Could you check a few things on this model? Use its own coordinates, in mm. Face numbers are marked on the shaded views. A direction names the side the tool comes from. Round coordinates to 2 decimals unless told otherwise and drop trailing zeros. Order: outer loops, then holes, each group sorted by start corner. A loop starts at its lowest first (then second) coordinate and runs counter-clockwise, first axis right, second up. Notation, with made-up numbers: (35.5, 49.25) - (44.5, 49.25) arc R28 cw to (44.5, 83.25) - close; hole circle Ø5 at (86.25, 89.25). An arc over 180 degrees is marked (long way). Return JSON: item names as keys, results as strings. Group by question number.
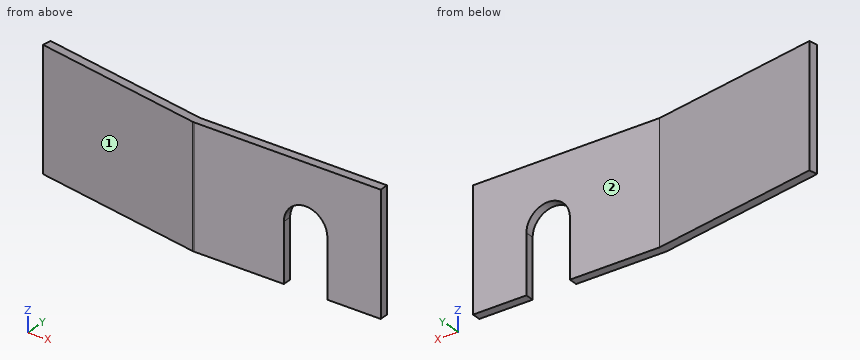
from build123d import *

# Parameters (mm, degrees)
F1_DEPTH      = 3
F3_DEPTH      = 21.6650813818
F3_DEPTH_BACK = 20.2457859941


with BuildPart() as f1:
    # F0 (on Front) → F1 (new body)
    with BuildSketch(Plane.XZ):
        with BuildLine():
            ThreePointArc((-7.5, 0), (0, 7.5), (7.5, 0))
            Line((7.5, 0), (7.5, -20.2457859941))
            Line((7.5, -20.2457859941), (25.9074462614, -20.2457859941))
            Line((25.9074462614, -20.2457859941), (25.9074462614, 21.6650813818))
            Line((25.9074462614, 21.6650813818), (-38.4318618068, 21.6650813818))
            Line((-38.4318618068, 21.6650813818), (-38.4318618068, -20.2457859941))
            Line((-38.4318618068, -20.2457859941), (-7.5, -20.2457859941))
            Line((-7.5, -20.2457859941), (-7.5, 0))
        make_face()
    extrude(amount=F1_DEPTH)

    # F2 (on Top) → F3 (join, two sides)
    with BuildSketch(Plane.XY) as f3_sk:
        with BuildLine():
            Line((-38.4318618068, -3), (-38.4318618068, 0))
            Line((-38.4318618068, 0), (-97.5203269875, 10.41889066))
            Line((-97.5203269875, 10.41889066), (-98.0412715205, 7.464467401))
            Line((-98.0412715205, 7.464467401), (-38.9528063398, -2.954423259))
            ThreePointArc((-38.9528063398, -2.954423259), (-38.693329035, -2.9885840943), (-38.4318618068, -3))
        make_face()
    extrude(amount=F3_DEPTH)
    extrude(f3_sk.sketch, amount=-F3_DEPTH_BACK)


solid = f1.part
1) If I drill on line 1 along Y through (x, z) = (18, 13.5); line 2 along Y through (x, z) = (-39.5, -15), over which ranges is the centre line in solid material (lowest first)? Write a range as from..to.
2) I want a section at B-B, the plane z = 18. List the corners of the cut face in (x, y) for me.
3) I want a section at D-D, the plane x = 0. List the corners of the cut face in (y, z) for me.
4) Will these pins go through, and if not, where does the flat tip stop? pin 1 (5 mm diameter, centred on x = -32.5, z = -1, fed in from +Y); pin 2 (1 mm diameter, centred on x = -80.5, y = 3, fed in from -Z).
5) For the marked faces 1 and 2, which set-ups out of +Z, -Z, +X, -X, +Y, -Y let a thin tool reach every point of the face, with its end or its side?
6) I want a section at C-C, the plane y = -1.25. List the corners of the cut face in (x, z) for me.
7) I want a section at A-A, the plane z = -17. List the corners of the cut face in (x, y) for me, plus the area to 3 significant figures.
Outcome:
{
 "1": {"line 1": "-3..0", "line 2": "-2.86..0.19"},
 "2": {"outline": "(-98.04, 7.46) - (-38.95, -2.95) arc R3 ccw to (-38.43, -3) - (25.91, -3) - (25.91, 0) - (-38.43, 0) - (-97.52, 10.42) - close"},
 "3": {"outline": "(-3, 7.5) - (0, 7.5) - (0, 21.67) - (-3, 21.67) - close"},
 "4": {"pin 1": "y = 0", "pin 2": "through"},
 "5": {"face 1": "+Z, -Z, -X, -Y", "face 2": "+Z, -Z, +X, +Y"},
 "6": {"outline": "(-48.62, -20.25) - (-7.5, -20.25) - (-7.5, 0) arc R7.5 cw to (7.5, 0) - (7.5, -20.25) - (25.91, -20.25) - (25.91, 21.67) - (-48.62, 21.67) - close"},
 "7": {"outline": "(-98.04, 7.46) - (-38.95, -2.95) arc R3 ccw to (-38.43, -3) - (-7.5, -3) - (-7.5, 0) - (-38.43, 0) - (-97.52, 10.42) - close; (7.5, -3) - (25.91, -3) - (25.91, 0) - (7.5, 0) - close", "area": "329 mm^2"}
}
